from build123d import *

# Parameters (mm, degrees)
BOSS_EXTRUDE1_DEPTH = 3
BOSS_EXTRUDE6_DEPTH = 22
CUT_EXTRUDE2_REACH  = 157.399
SKETCH23_R          = 1.5
FILLET2_R           = 1
SKETCH26_W          = 62.629754997
SKETCH26_H          = 21
BOSS_EXTRUDE8_DEPTH = 0.1
CUT_EXTRUDE4_REACH  = 155.098
SKETCH28_R          = 7


with BuildPart() as part:
    # Sketch1 → Boss-Extrude1 (new body)
    with BuildSketch(Plane.XY):
        with BuildLine():
            Line((0.088772672, 50.445513271), (0.088772672, 108.445513271))
            Line((0.088772672, 108.445513271), (20.088772672, 108.445513271))
            Line((20.088772672, 108.445513271), (20.088772672, 112.445513271))
            Line((20.088772672, 112.445513271), (40.088772672, 112.445513271))
            Line((40.088772672, 112.445513271), (40.088772672, 116.445513271))
            Line((40.088772672, 116.445513271), (60.088772672, 116.445513271))
            Line((60.088772672, 116.445513271), (60.088772672, 120.445513271))
            Line((60.088772672, 120.445513271), (80.088772672, 120.445513271))
            Line((80.088772672, 120.445513271), (80.088772672, 62.445513271))
            Line((80.088772672, 62.445513271), (95.696655206, 49.939754486))
            Line((95.696655206, 49.939754486), (79.719999866, 30))
            Line((79.719999866, 30), (79.719999866, 5))
            ThreePointArc((79.719999866, 5), (78.255533771, 1.464466094), (74.719999866, 0))
            Line((74.719999866, 0), (45.081340107, 0))
            Line((45.081340107, 0), (12.090244869, 0))
            ThreePointArc((12.090244869, 0), (10.402431062, 0.519821669), (9.299525382, 1.899143631))
            ThreePointArc((9.299525382, 1.899143631), (2.402932305, 25.737613543), (0.088772672, 50.445513271))
        make_face()
    extrude(amount=-BOSS_EXTRUDE1_DEPTH)

    # Sketch19 → Boss-Extrude6 (add)
    with BuildSketch(Plane.XY):
        with BuildLine():
            Line((45.081340107, 0), (12.090244869, 0))
            ThreePointArc((12.090244869, 0), (10.402431062, 0.519821669), (9.299525382, 1.899143631))
            ThreePointArc((9.299525382, 1.899143631), (2.402932305, 25.737613543), (0.088772672, 50.445513271))
            Line((0.088772672, 50.445513271), (3.088772672, 50.445513271))
            ThreePointArc((3.088772672, 50.445513271), (3.16127999, 48.288360754), (3.269039313, 46.132681692))
            Line((3.269039313, 46.132681692), (7.269039313, 46.132681692))
            Line((7.269039313, 46.132681692), (7.269039313, 41.132681692))
            Line((7.269039313, 41.132681692), (3.810920964, 39.61137507))
            ThreePointArc((3.810920964, 39.61137507), (6.552384593, 23.576295262), (11.244934046, 8.000050948))
            Line((11.244934046, 8.000050948), (18.244934046, 8.000050948))
            Line((18.244934046, 8.000050948), (18.244934046, 2.984064914))
            Line((18.244934046, 2.984064914), (45.23554431, 2.984064914))
            Line((45.23554431, 2.984064914), (69.874178677, 2.984064914))
            Line((69.874178677, 2.984064914), (69.874178677, 7.984064914))
            Line((69.874178677, 7.984064914), (76.874178677, 7.984064914))
            Line((76.874178677, 7.984064914), (76.933259672, 26.52199324))
            Line((76.933259672, 26.52199324), (79.719999866, 30))
            Line((79.719999866, 30), (79.719999866, 5))
            ThreePointArc((79.719999866, 5), (78.255533771, 1.464466094), (74.719999866, 0))
            Line((74.719999866, 0), (45.081340107, 0))
        make_face()
    extrude(amount=-BOSS_EXTRUDE6_DEPTH)

    # Sketch23 → Cut-Extrude2 (cut, up to next)
    with BuildSketch(Plane(origin=(0, 0, -22), x_dir=(-1, 0, 0), z_dir=(0, 0, -1)), mode=Mode.PRIVATE) as cut_extrude2_sk1:
        with Locations((-4.269039313, 43.132681692)):
            Circle(SKETCH23_R)
    cut_extrude2_tool1 = extrude(cut_extrude2_sk1.sketch, amount=-CUT_EXTRUDE2_REACH, mode=Mode.PRIVATE) & part.part
    # Sketch23 → Cut-Extrude2 (cut, up to next)
    with BuildSketch(Plane(origin=(0, 0, -22), x_dir=(-1, 0, 0), z_dir=(0, 0, -1)), mode=Mode.PRIVATE) as cut_extrude2_sk2:
        with Locations((-14.244934046, 4.500050948)):
            Circle(SKETCH23_R)
    cut_extrude2_tool2 = extrude(cut_extrude2_sk2.sketch, amount=-CUT_EXTRUDE2_REACH, mode=Mode.PRIVATE) & part.part
    # Sketch23 → Cut-Extrude2 (cut, up to next)
    with BuildSketch(Plane(origin=(0, 0, -22), x_dir=(-1, 0, 0), z_dir=(0, 0, -1)), mode=Mode.PRIVATE) as cut_extrude2_sk3:
        with Locations((-73.874178677, 4.484064914)):
            Circle(SKETCH23_R)
    cut_extrude2_tool3 = extrude(cut_extrude2_sk3.sketch, amount=-CUT_EXTRUDE2_REACH, mode=Mode.PRIVATE) & part.part
    add(cut_extrude2_tool1.solids().sort_by_distance((4.269039, 43.132682, -22))[0], mode=Mode.SUBTRACT)
    add(cut_extrude2_tool2.solids().sort_by_distance((14.244934, 4.500051, -22))[0], mode=Mode.SUBTRACT)
    add(cut_extrude2_tool3.solids().sort_by_distance((73.874179, 4.484065, -22))[0], mode=Mode.SUBTRACT)

    # Fillet2
    fillet2_edges = [part.edges().sort_by_distance(p)[0] for p in [
        (78.255533771, 1.464466094, 0),
        (43.405122367, 0, 0),
        (10.402431062, 0.519821669, 0),
        (2.402932305, 25.737613543, 0),
        (0.088772672, 79.445513271, 0),
        (10.088772672, 108.445513271, 0),
        (20.088772672, 110.445513271, 0),
        (30.088772672, 112.445513271, 0),
        (40.088772672, 114.445513271, 0),
        (50.088772672, 116.445513271, 0),
        (60.088772672, 118.445513271, 0),
        (70.088772672, 120.445513271, 0),
        (80.088772672, 91.445513271, 0),
        (87.892713939, 56.192633878, 0),
        (87.708327536, 39.969877243, 0),
        (79.719999866, 17.5, 0),
    ]]
    fillet(fillet2_edges, radius=FILLET2_R)

    # Sketch26 → Boss-Extrude8 (add)
    with BuildSketch(Plane.XZ):
        with Locations((43.405122368, -11.5)):
            Rectangle(SKETCH26_W, SKETCH26_H)
    extrude(amount=BOSS_EXTRUDE8_DEPTH)

    # Sketch28 → Cut-Extrude4 (cut, up to next)
    with BuildSketch(Plane(origin=(0, 2.984064914, 0), x_dir=(1, 0, 0), z_dir=(0, 1, 0)), mode=Mode.PRIVATE) as cut_extrude4_sk1:
        with Locations(Location((44.059556361, 12.5, 0), (0, 0, 180))):
            Circle(SKETCH28_R)
    cut_extrude4_tool1 = extrude(cut_extrude4_sk1.sketch, amount=-CUT_EXTRUDE4_REACH, mode=Mode.PRIVATE) & part.part
    add(cut_extrude4_tool1.solids().sort_by_distance((44.059556, 2.984065, -12.5))[0], mode=Mode.SUBTRACT)


solid = part.part
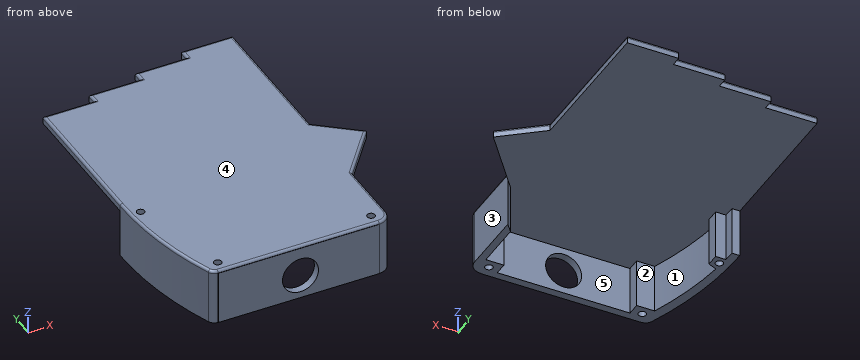
Verification items for the finished model (mm, model axes). Face numbers are marked on the shaded views. A direction names the side the tool comes from. Give positions to 0.01 mm unless a question says otherwise; leave off trailing zeros. Loops run counter-clockwise (first coordinate to the right, second up) from the corner with the lowest first, then second, coordinate; pieces in that order, holes last. Notation, with made-up numbers: (2.5, -35.5) - (31.5, -35.5) arc R23 cw to (31.5, -16.5) - close; hole circle Ø8 at (10.5, -29.5). An arc over 180 degrees is marked (long way). Write item = value, one per line. Start each with the question number.
Q1. Cross-section at D-D, the plane x = 35. Enter the section's corners in (y, z), and give its area (3 significant figures).
Q2. Tool access check on the marked faces 4 and 5. Record the directions out of +Z, -Z, +X, -X, +Y, -Y that give a thin tool (end or side, any length) a straight path to the whole face; none if there is none.
Q3. Cross-section at A-A, the plane z = -12.5. Enter the section's corners in (x, y).
Q4. Cross-section at B-B, the plane y = 77.5. Enter the section's corners in (x, z), and give its area (3 significant figures).
Q5. Cross-section at C-C, the plane x = 65. Enter the section's corners in (y, z).
Q6. Mould release check, pull along Y, two halves, no side actions. Record for the marked faces 1, 2 and 3: released by +Y, released by -Y, zero draft, split by the parting line, or undercut.
Q7. Thickness scan on line 1 (X direction, y = 85, z = -2); line 2 (Z direction, x = 66, y = 70.5); line 3 (Y direction, x = 56, z = -14.5). Record the ranges inside material, lowest first.
Q8. Depth check by flat-ended pin: P1, Ø1.5, axis at y = 6.5, z = -10.5, coming from the -X side; P2, Ø8, axis at y = 16, z = -12.5, coming from the -X side; P3, Ø1.5, axis at x = 1.5, z = -12, coming from the +Y side; P4, Ø5, axis at x = 14.24, y = 4.5, coming from the +Z side. Enter the tip coordinate at first touch or a pass-through.
Answer key:
q1.outline = (-0.1, -22) - (2.98, -22) - (2.98, -3) - (112.45, -3) - (112.45, -1) arc R1 ccw to (111.45, 0) - (1, 0) arc R1 ccw to (0, -1) - (-0.1, -1) - close
q1.area = 396 mm^2
q2.face_4 = +Z, +X, -X, +Y, -Y
q2.face_5 = -Z, +Y
q3.outline = (0.09, 50.45) arc R132.04 ccw to (9.3, 1.9) arc R3 ccw to (12.09, 0) - (12.09, -0.1) - (37.06, -0.1) - (37.06, 2.98) - (18.24, 2.98) - (18.24, 8) - (11.24, 8) arc R132.04 cw to (3.81, 39.61) - (7.27, 41.13) - (7.27, 46.13) - (3.27, 46.13) arc R132.04 cw to (3.09, 50.45) - close; (51.06, -0.1) - (74.72, -0.1) - (74.72, 0) arc R5 ccw to (79.72, 5) - (79.72, 30) - (76.93, 26.52) - (76.87, 7.98) - (69.87, 7.98) - (69.87, 2.98) - (51.06, 2.98) - close; hole circle Ø3 at (4.27, 43.13); hole circle Ø3 at (14.24, 4.5); hole circle Ø3 at (73.87, 4.48)
q4.outline = (0.09, -3) - (80.09, -3) - (80.09, -1) arc R1 ccw to (79.09, 0) - (1.09, 0) arc R1 ccw to (0.09, -1) - close
q4.area = 240 mm^2
q5.outline = (-0.1, -22) - (2.98, -22) - (2.98, -3) - (120.45, -3) - (120.45, -1) arc R1 ccw to (119.45, 0) - (1, 0) arc R1 ccw to (0, -1) - (-0.1, -1) - close
q6.face_1 = undercut
q6.face_2 = released by +Y
q6.face_3 = zero draft
q7.line_1 = 0.09 to 80.09
q7.line_2 = -3 to 0
q7.line_3 = -0.1 to 2.98
q8.P1 = 7.32
q8.P2 = 3.62
q8.P3 = 50.45
q8.P4 = 0
